For this review, take the finished solid that the model builds, in its own axes (mm). Face numbers are marked on the shaded views. A direction names the side the tool comes from. Give positions to 0.01 mm unless a question says otherwise; leave off trailing zeros. Order: outer loops, then holes, each group sorted by start corner. A loop starts at its lowest first (then second) coordinate and runs counter-clockwise, first axis right, second up. Notation, with made-up numbers: (18.25, -2.75) - (76.25, -2.75) arc R22 cw to (76.25, 19.25) - close; hole circle Ø9 at (63, -24.75). An arc over 180 degrees is marked (long way). Use a Markdown table: item, result. Add a question column.
1) We need section B-B on x = 2.5. Write out the cut boundary in (y, z), then the cut area to 3 significant figures.
2) Mouldability with a two-part tool opening along Y and no side actions: class the marked faces 1, 2, 3 and 4 as released by +Y, released by -Y, zero draft, split by the parting line, or undercut.
3) Clearance check with flat-ended pins moving along their axes: P1, Ø15, axis at x = 12, y = -2.5, coming from the -Z side; P2, Ø5, axis at x = 9, y = 10, coming from the -Z side; P3, Ø1.5, axis at y = -8.5, z = 1, coming from the +X side. State where each tip first meets the part, or that it passes through.
4) Machinability: for the marked faces 5, 6 and 7, which of the approach directions +Z, -Z, +X, -X, +Y, -Y give a long, thin tool a straight path to every point of the face, cutting with its end or side? Answer none if there is none.
5) Wall thickness on L1, parallel to X at y = -6.5, z = 0; L2, parallel to X at y = -6, z = 0; L3, parallel to X at y = 2.5, z = 0: over which ranges is each line inside the solid? List them lowest first.
6) We need section A-A on z = 0. Give the number of separate pieces and of enclosed holes in the cut face, then the cut area to 3 significant figures.
7) We need section C-C on z = -3.75. Write out the cut boundary in (x, y), then the cut area to 3 significant figures.
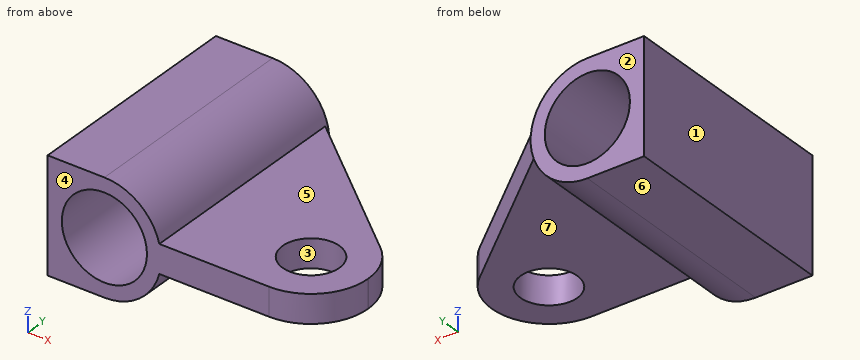
```python
from build123d import *

# Parameters (mm, degrees)
SKETCH1_R                = 6.35
SKETCH1_R_2              = 4.7625
BOSS_EXTRUDE1_DEPTH      = 12.7
BOSS_EXTRUDE2_DEPTH      = 1.5875
SKETCH3_R                = 3.175
CUT_EXTRUDE1_DEPTH       = 29.941304933
BOSS_EXTRUDE3_REACH      = 36.202
BOSS_EXTRUDE3_END_RADIUS = 6.35
SKETCH4_W                = 12.7
SKETCH4_H                = 25.4


with BuildPart() as part:
    # Sketch1 → Boss-Extrude1 (new, symmetric)
    with BuildSketch(Plane(origin=(0, 0, 0), x_dir=(1, 0, 0), z_dir=(0, 1, 0))):
        with Locations(Location((0, 0, 0), (0, 0, 270))):
            Circle(SKETCH1_R)
        with Locations(Location((0, 0, 0), (0, 0, 270))):
            Circle(SKETCH1_R_2, mode=Mode.SUBTRACT)
    extrude(amount=BOSS_EXTRUDE1_DEPTH, both=True)

    # Sketch2 → Boss-Extrude2 (add, symmetric)
    with BuildSketch(Plane.XY):
        with BuildLine():
            Line((5.715, -12.7), (18.415, -12.7))
            ThreePointArc((18.415, -12.7), (22.905128061, -10.840128061), (24.765, -6.35))
            Line((24.765, -6.35), (24.765, -6.245901603))
            ThreePointArc((24.765, -6.245901603), (24.170054448, -3.562275641), (22.496701322, -1.381519389))
            Line((22.496701322, -1.381519389), (5.715, 12.7))
            Line((5.715, 12.7), (5.715, -12.7))
        make_face()
    extrude(amount=BOSS_EXTRUDE2_DEPTH, both=True)

    # Sketch3 → Cut-Extrude1 (cut, through all)
    with BuildSketch(Plane.XY.offset(1.5875)):
        with Locations((18.415, -6.35)):
            Circle(SKETCH3_R)
    extrude(amount=-CUT_EXTRUDE1_DEPTH, mode=Mode.SUBTRACT)

    # Boss-Extrude3: up to this cylinder (the profile starts outside it)
    boss_extrude3_end = Plane(origin=(0, 0, 0), z_dir=(0, -1, 0)) * Cylinder(BOSS_EXTRUDE3_END_RADIUS, 86.104, mode=Mode.PRIVATE)
    # Sketch4 → Boss-Extrude3 (add, up to the surface)
    with BuildSketch(Plane.ZY.offset(6.35), mode=Mode.PRIVATE) as boss_extrude3_sk1:
        Rectangle(SKETCH4_W, SKETCH4_H)
    boss_extrude3_tool1 = extrude(boss_extrude3_sk1.sketch, amount=-BOSS_EXTRUDE3_REACH, mode=Mode.PRIVATE) - boss_extrude3_end
    add(boss_extrude3_tool1.solids().sort_by_distance((-6.35, 0, 0))[0])
    add(boss_extrude3_tool1.solids().sort_by_distance((-6.35, 0, 0))[1])


solid = part.part
```
Checked values:
| question | item | result |
|---|---|---|
| 1 | outline | (-12.7, -5.84) - (12.7, -5.84) - (12.7, -4.05) - (-12.7, -4.05) - close; (-12.7, 4.05) - (12.7, 4.05) - (12.7, 5.84) - (-12.7, 5.84) - close |
| 1 | area | 90.6 mm² |
| 2 | face 1 | zero draft |
| 2 | face 2 | released by +Y |
| 2 | face 3 | undercut |
| 2 | face 4 | released by -Y |
| 3 | P1 | z = -4.48 |
| 3 | P2 | z = -1.59 |
| 3 | P3 | x = 24.61 |
| 4 | face 5 | +Z, +X, +Y, -Y |
| 4 | face 6 | -Z, +X, -X, +Y, -Y |
| 4 | face 7 | -Z, +X, +Y, -Y |
| 5 | L1 | -6.35 to -4.76, 4.76 to 15.24, 21.59 to 24.76 |
| 5 | L2 | -6.35 to -4.76, 4.76 to 15.26, 21.57 to 24.76 |
| 5 | L3 | -6.35 to -4.76, 4.76 to 17.87 |
| 6 | separate pieces | 2 |
| 6 | enclosed holes | 1 |
| 6 | area | 355 mm² |
| 7 | outline | (-6.35, -12.7) - (-2.94, -12.7) - (-2.94, 12.7) - (-6.35, 12.7) - close; (2.94, -12.7) - (5.12, -12.7) - (5.12, 12.7) - (2.94, 12.7) - close |
| 7 | area | 142 mm² |
